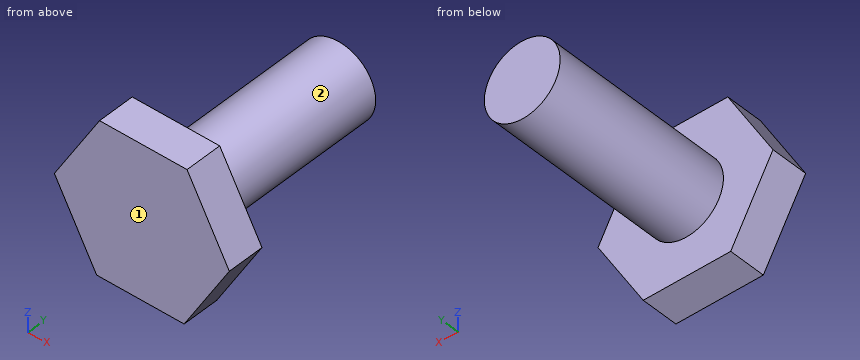
from build123d import *

# Parameters (mm, degrees)
SKETCH1_R           = 2
BOSS_EXTRUDE1_DEPTH = 10
BOSS_EXTRUDE4_DEPTH = 2


with BuildPart() as part:
    # Sketch1 → Boss-Extrude1 (new body)
    with BuildSketch(Plane(origin=(0, 0, 0), x_dir=(1, 0, 0), z_dir=(0, 1, 0))):
        with Locations((-18.876405997, -12.710678642)):
            Circle(SKETCH1_R)
    extrude(amount=BOSS_EXTRUDE1_DEPTH)

    # Sketch4 → Boss-Extrude4 (add)
    with BuildSketch(Plane.XZ):
        Polygon((-16.490145939, 16.665308368), (-21.108085773, 16.754555336), (-23.494345831, 12.79992561), (-21.262666056, 8.756048917), (-16.644726221, 8.666801949), (-14.258466163, 12.621431674), align=None)
    extrude(amount=BOSS_EXTRUDE4_DEPTH)


solid = part.part
Here's how the part is built. I have some questions about the finished solid (model axes, mm). Face numbers are marked on the shaded views. A direction names the side the tool comes from. Round coordinates to 2 decimals unless told otherwise and drop trailing zeros. Loops run counter-clockwise (first coordinate to the right, second up) from the corner with the lowest first, then second, coordinate; pieces in that order, holes last. Notation, with made-up numbers: (81, 59.25) - (100, 59.25) arc R20 ccw to (100, 88.25) - close; hole circle Ø8 at (23, 76). An arc over 180 degrees is marked (long way). One line per question, with ' | ' between items. Start each with the question number.
Q1. I want a section at C-C (y = -1). Write out the boundary of the cut face in (x, z).
Q2. I want a section at A-A (z = 14.25). Write out the boundary of the cut face in (x, y), then the cut area to 3 significant figures.
Q3. I want a section at B-B (x = -18). Write out the boundary of the cut face in (y, z).
Q4. Will these pins go through, and if not, where does the flat tip stop? pin 1 (3 mm diameter, centred on y = 4.5, z = 12, fed in from -X); pin 2 (3 mm diameter, centred on x = -22, z = 12.5, fed in from +Y); pin 3 (1 mm diameter, centred on x = -16.5, z = 14.5, fed in from +Y); pin 4 (3 mm diameter, centred on y = 7, z = 13, fed in from +X).
Q5. For the marked faces 1 and 2, which set-ups out of +Z, -Z, +X, -X, +Y, -Y let a thin tool reach every point of the face, with its end or its side?
Q6. Please list where these lines run through material, in increasing order: line 1 (Y direction, x = -16.5, z = 12.25); line 2 (Z direction, x = -19, y = 0.5); line 3 (X direction, y = 3.25, z = 12.25). Write a range as [from, to].
Q7. I want a section at D-D (x = -22). Write out the boundary of the cut face in (y, z).
Response values:
1) outline: (-23.49, 12.8) - (-21.26, 8.76) - (-16.64, 8.67) - (-14.26, 12.62) - (-16.49, 16.67) - (-21.11, 16.75) - close
2) outline: (-22.62, -2) - (-15.16, -2) - (-15.16, 0) - (-17.6, 0) - (-17.6, 10) - (-20.15, 10) - (-20.15, 0) - (-22.62, 0) - close | area: 40.5 mm²
3) outline: (-2, 8.69) - (0, 8.69) - (0, 10.91) - (10, 10.91) - (10, 14.51) - (0, 14.51) - (0, 16.69) - (-2, 16.69) - close
4) pin 1: stops at x = -20.88 | pin 2: stops at y = 10 | pin 3: stops at y = 0 | pin 4: stops at x = -16.88
5) face 1: +Z, -Z, +X, -X, -Y | face 2: +Y
6) line 1: y = [-2, 0] | line 2: z = [10.71, 14.71] | line 3: x = [-20.82, -16.93]
7) outline: (-2, 10.09) - (0, 10.09) - (0, 15.28) - (-2, 15.28) - close
